Autodesk Inventor part; units mm, degrees
ref_plane "YZ Plane" through (0, 0, 0) normal (1, 0, 0) x (0, 1, 0)
ref_plane "XZ Plane" through (0, 0, 0) normal (0, 1, 0) x (-1, 0, 0)
ref_plane "XY Plane" through (0, 0, 0) normal (0, 0, 1) x (1, 0, 0)
sketch "Sketch1" plane through (0, 0, 0) normal (0, 0, 1) x (1, 0, 0)
  line L0 (-14, 12.5) -> (14, 12.5)
  line L1 (14, 12.5) -> (14, -12.5)
  line L2 (14, -12.5) -> (-14, -12.5)
  line L3 (-14, -12.5) -> (-14, 12.5)
  circle A0 centre (0, 6.5) radius 8
  line L4 (-8, 12.5) -> (-8, 6.5)
  line L5 (-8, 1.1823) -> (-8, 1.3302)
  line L6 (8, 12.5) -> (8, 6.5)
  point P0 (0, 0)
  point P1 (-14, 0)
  point P2 (0, 12.5)
  point P3 (5.2915, 12.5)
  point P4 (-5.2915, 12.5)
  dimension "d0" = 28
  dimension "d1" = 25
  dimension "d2" = 16
  dimension "d4" = 11
extrude "Extrusion1" add sketch "Sketch1" along normal blind 2 contours L0 L4 A0 L6 L1 L2 L3
chamfer "Chamfer2" distance 2 angle 45 2 edges at (-8, 12.5, 1) (8, 12.5, 1)
properties part number "0008-10-058"
Read the model definition and answer for the solid it produces. Units are mm, in the model's axes. A direction names the side the tool comes from. Give positions to 0.01 mm unless a question says otherwise; leave off trailing zeros. Write each loop counter-clockwise with the first axis right and the second up, starting at its lowest first coordinate (ties: lowest second). Pieces come first, ordered by that corner, then holes. Notation, with made-up numbers: (12.5, -34) - (53.5, -34) arc R27 ccw to (53.5, -2) - close; hole circle Ø5 at (40, -24.75). An arc over 180 degrees is marked (long way). Use CSV: the item, a comma, the result in double quotes. Start each with the question number.
(1) Find section B-B (z = 0.3). Give the vertices of the cut face in (x, y).
(2) Determine the mould class of faces 3 (the flat face through (0, -3, 2)), 4 (the flat face through (-8, 9, 1)), 5 (the flat face through (-14, 0, 1)) for opening direction X: +X half, -X half, draft (parallel to the pull), parting line (faces both ways), or undercut.
(3) Find section C-C (x = 0). Give the vertices of the cut face in (y, z), plus the area to 3 significant figures.
(4) Consider line 1 along X through (y, z) = (6.5, 0.65); line 2 along X through (y, z) = (1.5, 1.4) (3 decimals); line 3 along Y through (x, z) = (3, 1.1). Determine where each line is inside the solid, lowest interval first.
(5) For faces 1 (the flat face through (8, 9, 1)), 2 (the flat face through (-12, 12.5, 1)), determine the directions among +Z, -Z, +X, -X, +Y, -Y from which every point of the face is accessible in a straight line to the end or side of a thin tool.
(6) Find section A-A (y = 7). Give the vertices of the cut face in (x, z).
Findings below:
1,outline,"(-14, -12.5) - (14, -12.5) - (14, 12.5) - (10, 12.5) - (8, 10.5) - (8, 6.5) arc R8 cw to (-8, 6.5) - (-8, 10.5) - (-10, 12.5) - (-14, 12.5) - close"
2,face 3,"draft"
2,face 4,"undercut"
2,face 5,"-X half"
3,outline,"(-12.5, 0) - (-1.5, 0) - (-1.5, 2) - (-12.5, 2) - close"
3,area,"22.0 mm2"
4,line 1,"-14 to -8, 8 to 14"
4,line 2,"-14 to -6.245, 6.245 to 14"
4,line 3,"-12.5 to -0.92"
5,face 1,"+Z, -Z, +Y"
5,face 2,"+Z, -Z, +X, -X, +Y"
6,outline,"(-14, 0) - (-8, 0) - (-8, 2) - (-14, 2) - close; (8, 0) - (14, 0) - (14, 2) - (8, 2) - close"
